Autodesk Inventor part; units mm, degrees
ref_plane "Płaszczyzna konstrukcyjna1" through (117.8756, 33, 145) normal (0, 0, 1) x (-1, 0, 0)
ref_plane "Płaszczyzna konstrukcyjna4" through (117.8756, 33, 72.5) normal (0, 0, -1) x (-1, 0, 0)
ref_plane "Płaszczyzna konstrukcyjna6" through (0, 0, 72.5) normal (0, 0, 1) x (1, 0, 0)
sketch "Szkic1" plane through (0, 0, 0) normal (0, 0, 1) x (1, 0, 0)
  arc A0 (0, 35) -> (0, -35) centre (0, 0) ccw construction
  line L0 (0, 35) -> (390, 35) construction
  line L1 (0, -35) -> (390, -35) construction
  arc A1 (390, -35) -> (390, 35) centre (390, 0) ccw construction
  circle A2 centre (0, 0) radius 4.5
  circle A3 centre (390, 0) radius 4.5
  line L2 (130, 35) -> (130, 10) construction
  line L3 (260, 35) -> (260, 10) construction
  circle A4 centre (130, 10) radius 25 construction
  circle A5 centre (260, 10) radius 25 construction
  circle A6 centre (130, 10) radius 4.5
  circle A7 centre (260, 10) radius 4.5
  circle A8 centre (0, 0) radius 35 construction
  circle A9 centre (390, 0) radius 35 construction
  line L4 (117.8756, 33) -> (31.8551, 33)
  line L5 (375.6125, 33) -> (272.1244, 33)
  line L6 (247.8756, 33) -> (142.1244, 33)
  line L7 (31.8551, 31) -> (114.6703, 31)
  line L8 (145.3297, 31) -> (244.6703, 31)
  line L9 (275.3297, 31) -> (371.697, 31)
  arc A10 (375.6125, 33) -> (371.697, 31) centre (390, 0) ccw
  arc A11 (117.8756, 33) -> (114.6703, 31) centre (130, 10) ccw
  arc A12 (145.3297, 31) -> (142.1244, 33) centre (130, 10) ccw
  arc A13 (247.8756, 33) -> (244.6703, 31) centre (260, 10) ccw
  arc A14 (275.3297, 31) -> (272.1244, 33) centre (260, 10) ccw
  line L10 (31.8551, 14.5) -> (31.8551, 35) construction
  line L11 (31.8551, 33) -> (31.8551, 31)
  line L12 (260, 10) -> (260, 0)
  line L13 (130, 10) -> (130, 0)
  point P0 (423.5971, -9.8098)
  dimension "d94" = 50
  dimension "d0" = 70
  dimension "d1" = 390
  dimension "d2" = 390
  dimension "d3" = 70
  dimension "d4" = 9
  dimension "d5" = 9
  dimension "d10" = 25
  dimension "d11" = 25
  dimension "d12" = 9
  dimension "d13" = 9
  dimension "d14" = 130
  dimension "d15" = 260
  dimension "d24" = 2
  dimension "d25" = 2
  dimension "d26" = 2
  dimension "d27" = 1
  dimension "d95" = 2
extrude "Wyciągnięcie proste1" add sketch "Szkic1" along normal blind 145 contours A11 L7 L11 L4 | A10 L9 A14 L5 | A13 L8 A12 L6
ref_plane "Płaszczyzna konstrukcyjna1" through (117.8756, 33, 145) normal (0, 0, 1) x (-1, 0, 0)
sketch "Szkic3" plane through (117.8756, 33, 145) normal (0, 0, 1) x (-1, 0, 0)
  circle A0 centre (117.8756, 33) radius 4.5
  arc A1 (133.7659, 28.5) -> (133.7659, 37.5) centre (133.7659, 33) ccw
  arc A2 (98.6659, 37.5) -> (98.6659, 28.5) centre (98.6659, 33) ccw
  line L0 (133.7659, 28.5) -> (98.6659, 28.5)
  line L1 (98.6659, 37.5) -> (133.7659, 37.5)
  line L2 (98.6659, 18.5) -> (133.7659, 18.5)
  arc A3 (133.7659, 18.5) -> (133.7659, 47.5) centre (133.7659, 33) ccw
  line L3 (133.7659, 47.5) -> (98.6659, 47.5)
  line L4 (86.0205, 18.5) -> (86.0205, -2) construction
  line L5 (98.6659, 18.5) -> (86.0205, 18.5)
  line L6 (98.6659, 47.5) -> (86.0205, 47.5)
  line L7 (86.0205, 0) -> (86.0205, 2)
  line L8 (86.0205, 18.5) -> (86.0205, 0)
  line L9 (98.6659, 47.5) -> (98.6659, 81.8113)
  line L10 (98.6659, 81.8113) -> (-234.1244, 81.8113)
  line L11 (-157.4541, 2) -> (-253.8214, 2)
  line L12 (86.0205, 0) -> (86.0205, 2)
  line L13 (-257.7369, 0) -> (-154.2487, 0)
  line L14 (86.0205, 0) -> (-238.0399, 0)
  circle A4 centre (-272.1244, 33) radius 35 construction
  line L15 (-234.1244, 2) -> (-234.1244, 18.5)
  line L16 (-234.1244, 2) -> (-238.0399, 0)
  line L17 (-246.7694, 47.5) -> (-246.7694, 81.8113)
  line L18 (-246.7694, 81.8113) -> (-234.1244, 81.8113)
  line L19 (-303.9795, 47.5) -> (-409.6259, 47.5) construction
  line L20 (-234.1244, 47.5) -> (-246.7694, 47.5)
  line L21 (-234.1244, 18.5) -> (-281.8694, 18.5)
  line L22 (-246.7694, 47.5) -> (-281.8694, 47.5)
  arc A5 (-281.8694, 47.5) -> (-281.8694, 18.5) centre (-281.8694, 33) ccw
  point P0 (-238.0399, 0)
  dimension "d33" = 9
  dimension "d34" = 9
  dimension "d35" = 10
  dimension "d36" = 47.7454
  dimension "d37" = 12.6455
  dimension "d38" = 12.6455
  dimension "d39" = 12.6455
  dimension "d40" = 0
  dimension "d64" = 47.745
  dimension "d93" = 16.5
extrude "Wyciągnięcie proste2" add sketch "Szkic3" along normal blind 4
ref_plane "Płaszczyzna konstrukcyjna4" through (117.8756, 33, 72.5) normal (0, 0, -1) x (-1, 0, 0)
mirror "Odbij2" about plane through (117.8756, 33, 72.5) normal (0, 0, -1) of "Wyciągnięcie proste2"
extrude "Wyciągnięcie proste4" cut sketch "Szkic1" along normal mid plane 10000 contours A6 | A7
sketch "Szkic8" plane through (0, 0, 145) normal (0, 0, 1) x (1, 0, 0)
  line L0 (352, 31) -> (371.697, 31)
  line L1 (352, 31) -> (355.9155, 33)
  line L2 (352, 31) -> (355.9155, 33)
  line L3 (375.6125, 33) -> (355.9155, 33)
  line L4 (355.9155, 33) -> (375.6125, 33)
  arc A0 (375.6125, 33) -> (371.697, 31) centre (390, 0) ccw
  line L5 (375.6125, 33) -> (371.697, 31)
  line L6 (352, 14.5) -> (352, 31)
  line L7 (371.697, 31) -> (352, 31)
  point P0 (0, 0)
  point P1 (352, -48.8113)
ref_plane "Płaszczyzna konstrukcyjna6" through (0, 0, 72.5) normal (0, 0, 1) x (1, 0, 0)
extrude "Wyciągnięcie proste5" cut sketch "Szkic8" along normal mid plane 1000 contours L1 L3 A0 L0
ref_plane "Płaszczyzna konstrukcyjna9" through (117.8756, 33, 149) normal (0, 0, 1) x (1, 0, 0)
sketch "Szkic12" plane through (117.8756, 33, 149) normal (0, 0, 1) x (1, 0, 0)
  line L0 (281.8694, -18.5) -> (234.1244, -18.5)
  arc A0 (281.8694, -47.5) -> (281.8694, -18.5) centre (281.8694, -33) ccw
  line L1 (246.7694, -47.5) -> (281.8694, -47.5)
  line L2 (246.7694, -81.8113) -> (246.7694, -47.5)
  line L3 (234.1244, -2) -> (234.1244, -81.8113)
  line L4 (-98.6659, -81.8113) -> (246.7694, -81.8113)
  point P0 (-117.8756, -33)
extrude "Wyciągnięcie proste7" cut sketch "Szkic12" against normal blind 17
extrude "Wyciągnięcie proste8" cut sketch "Szkic1" against normal blind 17 contours A3
ref_plane "Płaszczyzna konstrukcyjna10" through (117.8756, 33, 149) normal (0, 0, 1) x (1, 0, 0)
sketch "Szkic13" plane through (117.8756, 33, 149) normal (0, 0, 1) x (1, 0, 0)
  line L0 (234.1244, -81.8113) -> (234.1244, -2)
  line L1 (232.1244, -81.8113) -> (232.1244, -2)
  line L2 (234.1244, -2) -> (238.0399, 0)
  line L3 (238.0399, 0) -> (236.0399, 0)
  line L4 (238.0399, 0) -> (-86.0205, 0)
  line L5 (236.0399, 0) -> (232.1244, -2)
  line L6 (238.0399, 0) -> (234.1244, -2)
  line L7 (234.1244, -81.8113) -> (232.1244, -81.8113)
  line L8 (-98.6659, -81.8113) -> (246.7694, -81.8113)
  point P0 (-117.8756, -33)
  dimension "d70" = 2
  dimension "d71" = 2
extrude "Wyciągnięcie proste9" add sketch "Szkic13" along normal blind 17
ref_plane "Płaszczyzna konstrukcyjna11" through (117.8756, 33, 166) normal (0, 0, 1) x (1, 0, 0)
sketch "Szkic14" plane through (117.8756, 33, 166) normal (0, 0, 1) x (1, 0, 0)
  line L0 (232.1244, -81.8113) -> (234.1244, -81.8113)
  line L1 (-98.6659, -81.8113) -> (246.7694, -81.8113)
  line L2 (232.1244, -81.8113) -> (246.7694, -81.8113)
  line L3 (246.7694, -81.8113) -> (246.7694, -47.5)
  line L4 (246.7694, -81.8113) -> (246.7694, -47.5)
  line L5 (246.7694, -47.5) -> (281.8694, -47.5)
  line L6 (246.7694, -47.5) -> (281.8694, -47.5)
  line L7 (281.8694, -18.5) -> (234.1244, -18.5)
  line L8 (234.1244, -81.8113) -> (234.1244, -2)
  arc A0 (281.8694, -47.5) -> (281.8694, -18.5) centre (281.8694, -33) ccw
  circle A1 centre (272.1244, -33) radius 4.5
  line L9 (232.1244, -2) -> (232.1244, -81.8113)
  line L10 (236.0399, 0) -> (232.1244, -2)
  line L11 (238.0399, 0) -> (236.0399, 0)
  line L12 (234.1244, -2) -> (238.0399, 0)
  point P0 (-117.8756, -33)
extrude "Wyciągnięcie proste10" add sketch "Szkic14" along normal blind 4
ref_plane "Płaszczyzna konstrukcyjna12" through (364.645, -48.8113, -4) normal (0, 0, -1) x (-1, 0, 0)
sketch "Szkic15" plane through (364.645, -48.8113, -4) normal (0, 0, -1) x (-1, 0, 0)
  line L0 (332.7899, 63.3113) -> (322.7899, 63.3113)
  line L1 (322.7899, 63.3113) -> (322.7899, 34.3113)
  line L2 (322.7899, 34.3113) -> (332.7899, 34.3113)
  line L3 (332.7899, 34.3113) -> (332.7899, 63.3113)
  point P0 (364.645, 48.8113)
  dimension "d78" = 10
extrude "Wyciągnięcie proste11" add sketch "Szkic15" along normal blind 14.44
ref_plane "Płaszczyzna konstrukcyjna13" through (117.8756, 33, 149) normal (0, 0, 1) x (1, 0, 0)
sketch "Szkic16" plane through (117.8756, 33, 149) normal (0, 0, 1) x (1, 0, 0)
  line L0 (-86.0205, -18.5) -> (-133.7659, -18.5)
  line L1 (-86.0205, -47.5) -> (-76.0205, -47.5)
  line L2 (-86.0205, -18.5) -> (-76.0205, -18.5)
  line L3 (-76.0205, -18.5) -> (-76.0205, -47.5)
  line L4 (-76.0205, -47.5) -> (-86.0205, -47.5)
  line L5 (-86.0205, -47.5) -> (-86.0205, -18.5)
  point P0 (-117.8756, -33)
  point P1 (-86.0205, -47.5)
  dimension "d82" = 10
extrude "Wyciągnięcie proste12" add sketch "Szkic16" along normal blind 14.44
ref_plane "Płaszczyzna konstrukcyjna14" through (31.8551, -14.5, -4) normal (-1, 0, 0) x (0, 0, 1)
sketch "Szkic17" plane through (31.8551, -14.5, -4) normal (-1, 0, 0) x (0, 0, 1)
  line L0 (4, 0) -> (4, 29)
  line L1 (4, 19) -> (-14.44, 19)
  line L2 (-14.44, 29) -> (-14.44, 0)
  line L3 (4, 10) -> (0, 10)
  line L4 (4, 10) -> (-12.44, 10)
  line L5 (4, 18.5) -> (-12.44, 18.5)
  line L6 (-12.44, 18.5) -> (-4.44, 18.5)
  line L7 (-4.44, 18.5) -> (-4.44, 10.5)
  line L8 (-4.44, 10.5) -> (-12.44, 10.5)
  line L9 (-12.44, 10.5) -> (-12.44, 18.5)
  circle A0 centre (-8.44, 14.5) radius 2.5
  point P0 (4, 14.5)
  dimension "d86" = 9
  dimension "d87" = 0.5
  dimension "d88" = 8
  dimension "d89" = 8
  dimension "d90" = 5
extrude "Wyciągnięcie proste13" cut sketch "Szkic17" against normal through all contours A0
mirror "Odbij3" about plane through (117.8756, 33, 72.5) normal (0, 0, -1) of "Wyciągnięcie proste13"
ref_plane "Płaszczyzna konstrukcyjna15" through (364.645, -48.8113, -4) normal (0, 0, -1) x (-1, 0, 0)
sketch "Szkic19" plane through (364.645, -48.8113, -4) normal (0, 0, -1) x (-1, 0, 0)
  circle A0 centre (234.645, 58.8113) radius 4.5
  line L0 (234.645, 58.8113) -> (249.645, 58.8113)
  circle A1 centre (104.645, 58.8113) radius 4.5
  line L1 (104.645, 58.8113) -> (89.645, 58.8113)
  line L2 (89.645, 101.2973) -> (-85.4155, 101.2973)
  line L3 (-85.4155, 101.2973) -> (-85.4155, -16.8317)
  line L4 (-85.4155, -16.8317) -> (89.645, -16.8317)
  line L5 (89.645, -16.8317) -> (89.645, 101.2973)
  line L6 (249.645, 101.2973) -> (438.4161, 101.2973)
  line L7 (438.4161, 101.2973) -> (438.4161, -28.5413)
  line L8 (438.4161, -28.5413) -> (249.645, -28.5413)
  line L9 (249.645, -28.5413) -> (249.645, 101.2973)
  point P0 (364.645, 48.8113)
  dimension "d99" = 15
  dimension "d100" = 15
extrude "Wyciągnięcie proste14" cut sketch "Szkic19" along normal mid plane 682 contours L9 L6 L7 L8 | L5 L4 L3 L2
ref_plane "Płaszczyzna konstrukcyjna17" through (115, -48.8113, 149) normal (-1, 0, 0) x (0, 0, 1)
sketch "Szkic21" plane through (115, -48.8113, 149) normal (-1, 0, 0) x (0, 0, 1)
  line L0 (-149, 0) -> (-153, 0)
  line L1 (-151, 0) -> (-151, 15)
  line L2 (0, 0) -> (-4, 0)
  line L3 (-2, 0) -> (-2, 15)
  line L4 (0, 81.8113) -> (0, 0)
  line L5 (0, 81.8113) -> (-153, 81.8113)
  line L6 (-2, 81.8113) -> (-2, 66.8113)
  line L7 (-151, 81.8113) -> (-151, 66.8113)
  circle A0 centre (-151, 66.8113) radius 1
  circle A1 centre (-2, 66.8113) radius 1
  circle A2 centre (-2, 15) radius 1
  circle A3 centre (-151, 15) radius 1
  point P0 (-149, 48.8113)
  dimension "d112" = 15
  dimension "d113" = 15
  dimension "d114" = 15
  dimension "d115" = 2
  dimension "d116" = 2
  dimension "d117" = 2
  dimension "d118" = 2
extrude "Wyciągnięcie proste15" cut sketch "Szkic21" against normal blind 7
ref_plane "Płaszczyzna konstrukcyjna18" through (275, -48.8113, -4) normal (1, 0, 0) x (0, 0, -1)
sketch "Szkic22" plane through (275, -48.8113, -4) normal (1, 0, 0) x (0, 0, -1)
  circle A0 centre (-151, 66.8113) radius 1
  circle A1 centre (-151, 15) radius 1
  circle A2 centre (-2, 66.8113) radius 1
  line L0 (-4, 80.0481) -> (-4, 0)
  circle A3 centre (-2, 15) radius 1
  point P0 (-4, 48.8113)
extrude "Wyciągnięcie proste16" cut sketch "Szkic22" against normal blind 7
ref_plane "Płaszczyzna konstrukcyjna5" through (117.8756, 33, 72.5) normal (0, 0, -1) x (-1, 0, 0)
properties part number "Podstawacz2"
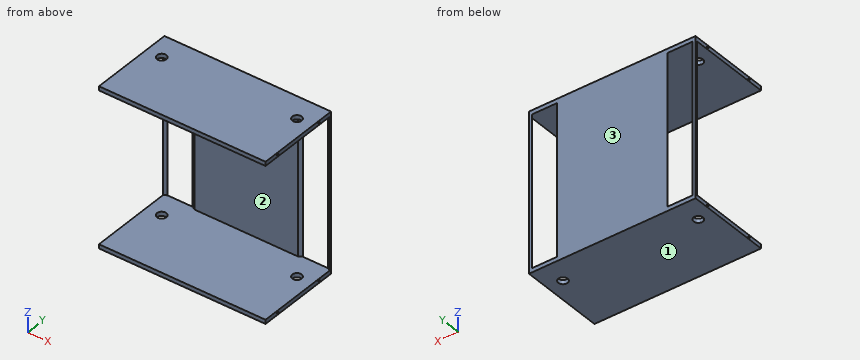
Check sheet for the modelled part. Datum: model origin and axes. Units: mm. Face numbers are marked on the shaded views. Give positions to 0.01 mm unless a question says otherwise; leave off trailing zeros. Write each loop counter-clockwise with the first axis right and the second up, starting at its lowest first coordinate (ties: lowest second). Pieces come first, ordered by that corner, then holes. Notation, with made-up numbers: (2, 12) - (48, 12) arc R28 cw to (48, 44) - close; hole circle Ø9 at (-24.5, 74). An arc over 180 degrees is marked (long way). Answer as a JSON object with one key per item and string values. Group by question number.
1) Sectioned sample at A-A (y = 10). Record the cut outline in (x, z).
2) Thickness scan on probe 1 along Y at (x, z) = (117, 147); probe 2 along Y at (x, z) = (130, 147.15); probe 3 along Z at (x, y) = (187.5, -29). Record the ranges inside material, lowest first. Write a range as from..to.
3) Sectioned sample at B-B (z = 39). Record the cut outline in (x, y) (1 decimal), then the cut area to 3 significant figures.
4) Sectioned sample at D-D (y = -15). Record the cut outline in (x, z), then the cut area to 3 significant figures.
5) Release check for a two-part mould opening along Z. For the marked faces 1, 2 and 3 record: pulls with the +Z half, pulls with the -Z half, needs draft (parallel to the pull), parting line crosses it, or undercut.
6) Depth check by flat-ended pin: P1, Ø3, axis at y = -33.81, z = -2, coming from the -X side; P2, Ø8, axis at x = 243.5, z = 83, coming from the -Y side; P3, Ø1.6, axis at y = 18, z = 147, coming from the -X side; P4, Ø1.8, axis at y = 18, z = 147, coming from the +X side. Enter the tip coordinate at first touch or a pass-through.
7) Sectioned sample at C-C (x = 260). Record the cut outline in (y, z), then the cut area to 3 significant figures.
Geometry results:
{
 "1": {"outline": "(115, -4) - (125.5, -4) - (125.5, 0) - (115, 0) - close; (115, 145) - (125.5, 145) - (125.5, 149) - (115, 149) - close; (134.5, -4) - (255.5, -4) - (255.5, 0) - (134.5, 0) - close; (134.5, 145) - (255.5, 145) - (255.5, 149) - (134.5, 149) - close; (264.5, -4) - (275, -4) - (275, 0) - (264.5, 0) - close; (264.5, 145) - (275, 145) - (275, 149) - (264.5, 149) - close"},
 "2": {"probe 1": "y = -48.81..-34.81, -32.81..17, 19..33", "probe 2": "y = -48.81..5.5, 14.5..33", "probe 3": "z = -4..0, 145..149"},
 "3": {"outline": "(115, 31.2) arc R26 cw to (117.9, 33) - (115, 33) - close; (142.1, 33) arc R26 cw to (145.3, 31) - (244.7, 31) arc R26 cw to (247.9, 33) - close; (272.1, 33) arc R26 cw to (275, 31.2) - (275, 33) - close", "area": "210 mm^2"},
 "4": {"outline": "(115, -4) - (275, -4) - (275, 0) - (115, 0) - close; (115, 145) - (275, 145) - (275, 149) - (115, 149) - close", "area": "1,280 mm^2"},
 "5": {"face 1": "pulls with the -Z half", "face 2": "undercut", "face 3": "needs draft"},
 "6": {"P1": "stops at x = 115", "P2": "stops at y = 31", "P3": "stops at x = 122", "P4": "stops at x = 268"},
 "7": {"outline": "(-48.81, -4) - (5.5, -4) - (5.5, 0) - (-48.81, 0) - close; (-48.81, 145) - (5.5, 145) - (5.5, 149) - (-48.81, 149) - close; (14.5, -4) - (33, -4) - (33, 0) - (14.5, 0) - close; (14.5, 145) - (33, 145) - (33, 149) - (14.5, 149) - close", "area": "582 mm^2"}
}
